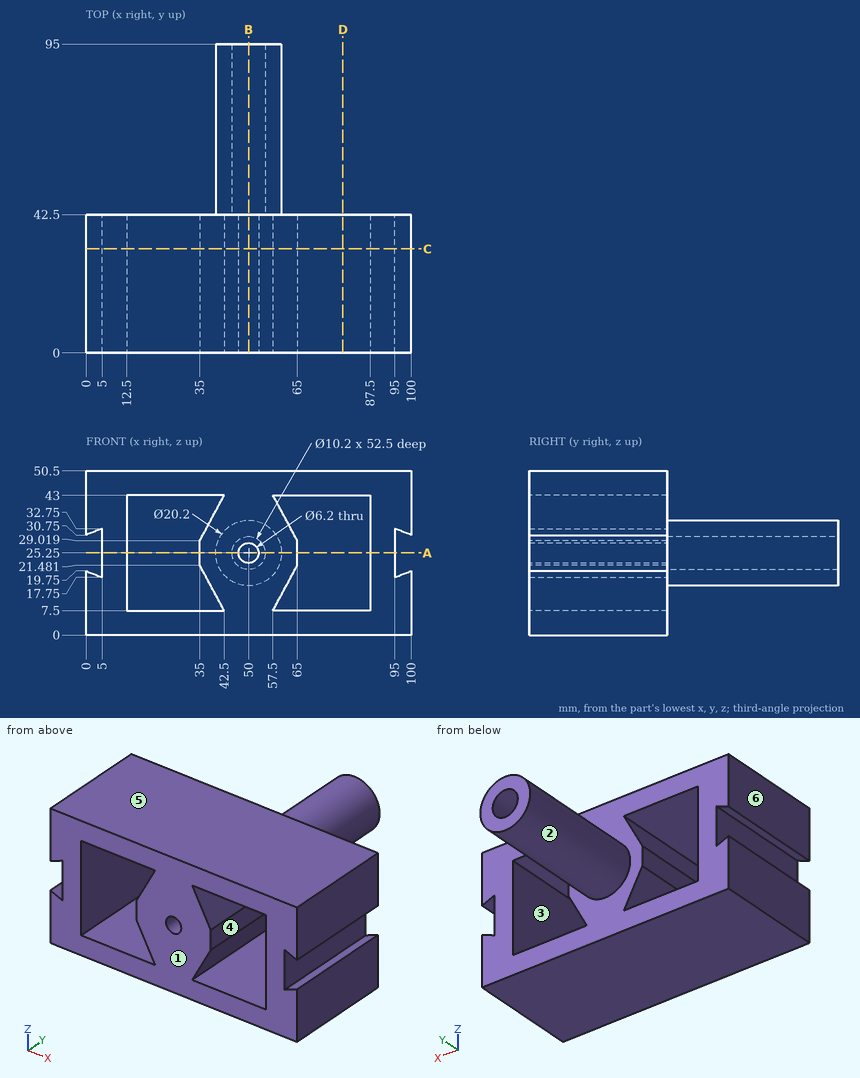
Study the drawing (mm; zero at the part's minimum x, y, z) and answer. A direction names the side the tool comes from. Round coordinates to 2 decimals unless told otherwise and drop trailing zeros. Loops run counter-clockwise (first coordinate to the right, second up) from the corner with the lowest first, then second, coordinate; pieces in that order, holes last. Notation, with made-up numbers: (43.25, 28) - (86.25, 28) arc R32 cw to (86.25, 59) - close; hole circle Ø1 at (75.5, 88). An arc over 180 degrees is marked (long way). Use one line per item in the form item = value. Start each with the question number.
1. Consider line 1 (Z direction, x = 21.5, y = 13.5); line 2 (X direction, y = 61, z = 25.25); line 3 (X direction, y = 31, z = 34). Determine where each line is inside the solid, lowest interval first. Write a range as [from, to].
2. The part is cut by section C-C on y = 32. Determine the outline of the cut face in (x, z), then the cut area to 3 significant figures.
3. For a pull along X with two mould halves and no side action, classify the marked faces 4, 5 and 6 as pulls with the +X half, pulls with the -X half, needs draft (parallel to the pull), parting line crosses it, or undercut.
4. Given pin 1 Ø8 at (y, z) = (65, 32) entering from +X; pin 2 Ø12 at (y, z) = (16.5, 27) entering from -X; pin 3 Ø4 at (y, z) = (19, 24.5) entering from -X; pin 4 Ø8.5 at (y, z) = (18, 26) entering from +X, each flat-ended and moving along its own axis, determine where each tip first touches the part or whether it passes through.
5. The part is cut by section B-B on x = 50. Determine the outline of the cut face in (y, z), then the cut area to 3 significant figures.
6. A tool of negligible diameter and unlimited length cuts with its end or side. For the marked faces 1, 2 and 3, from which of +Z, -Z, +X, -X, +Y, -Y can it reach the whole face along a straight path? Write none if from no direction.
7. The part is cut by section A-A on z = 25.25. Determine the outline of the cut face in (x, y).
8. The part is cut by section D-D on x = 79. Determine the outline of the cut face in (y, z).
Geometry check:
q1.line_1 = [0, 7.5], [43, 50.5]
q1.line_2 = [39.9, 44.9], [55.1, 60.1]
q1.line_3 = [0, 12.5], [37.67, 62.33], [87.5, 100]
q2.outline = (0, 0) - (100, 0) - (100, 19.75) - (95, 17.75) - (95, 32.75) - (100, 30.75) - (100, 50.5) - (0, 50.5) - (0, 30.75) - (5, 32.75) - (5, 17.75) - (0, 19.75) - close; hole (12.5, 7.5) - (42.5, 7.5) - (35, 21.48) - (35, 29.02) - (42.5, 43) - (12.5, 43) - close; hole circle Ø6.2 at (50, 25.25); hole (57.5, 7.5) - (87.5, 7.5) - (87.5, 43) - (57.5, 43) - (65, 29.02) - (65, 21.48) - close
q2.area = 3,080 mm^2
q3.face_4 = undercut
q3.face_5 = needs draft
q3.face_6 = pulls with the -X half
q4.pin_1 = 59.72
q4.pin_2 = 0
q4.pin_3 = 5
q4.pin_4 = 95
q5.outline = (0, 0) - (42.5, 0) - (42.5, 15.15) - (95, 15.15) - (95, 20.15) - (42.5, 20.15) - (42.5, 22.15) - (0, 22.15) - close; (0, 28.35) - (42.5, 28.35) - (42.5, 30.35) - (95, 30.35) - (95, 35.35) - (42.5, 35.35) - (42.5, 50.5) - (0, 50.5) - close
q5.area = 2,410 mm^2
q6.face_1 = +Z, -Z, +X, -X, -Y
q6.face_2 = +Y
q6.face_3 = +Y, -Y
q7.outline = (5, 0) - (12.5, 0) - (12.5, 42.5) - (5, 42.5) - close; (35, 0) - (46.9, 0) - (46.9, 42.5) - (44.9, 42.5) - (44.9, 95) - (39.9, 95) - (39.9, 42.5) - (35, 42.5) - close; (53.1, 0) - (65, 0) - (65, 42.5) - (60.1, 42.5) - (60.1, 95) - (55.1, 95) - (55.1, 42.5) - (53.1, 42.5) - close; (87.5, 0) - (95, 0) - (95, 42.5) - (87.5, 42.5) - close
q8.outline = (0, 0) - (42.5, 0) - (42.5, 7.5) - (0, 7.5) - close; (0, 43) - (42.5, 43) - (42.5, 50.5) - (0, 50.5) - close
